from build123d import *

# Parameters (mm, degrees)
SKETCH1_W           = 10.53028371
SKETCH1_H           = 7.9375
BOSS_EXTRUDE1_DEPTH = 6.35
BOSS_EXTRUDE2_DEPTH = 11.1125
SKETCH3_R           = 0.75
BOSS_EXTRUDE3_DEPTH = 3.5


with BuildPart() as part:
    # Sketch1 → Boss-Extrude1 (new body)
    with BuildSketch(Plane(origin=(0, 0, 0), x_dir=(1, 0, 0), z_dir=(0, 1, 0))):
        with BuildLine():
            Line((-5.265141855, 0), (-5.265141855, 7.9375))
            ThreePointArc((-5.265141855, 7.9375), (-8.392737967, 4.504173), (-9.525, 0))
            Line((-9.525, 0), (-5.265141855, 0))
        make_face()
        with BuildLine():
            Line((-5.265141855, -7.9375), (-5.265141855, 0))
            Line((-5.265141855, 0), (-9.525, 0))
            ThreePointArc((-9.525, 0), (-8.392737967, -4.504173), (-5.265141855, -7.9375))
        make_face()
        with Locations((0, -3.96875)):
            Rectangle(SKETCH1_W, SKETCH1_H)
        with BuildLine():
            ThreePointArc((9.525, 0), (8.392737967, 4.504173), (5.265141855, 7.9375))
            Line((5.265141855, 7.9375), (5.265141855, 0))
            Line((5.265141855, 0), (9.525, 0))
        make_face()
        with BuildLine():
            Line((9.525, 0), (5.265141855, 0))
            Line((5.265141855, 0), (5.265141855, -7.9375))
            ThreePointArc((5.265141855, -7.9375), (8.392737967, -4.504173), (9.525, 0))
        make_face()
        with Locations((0, 3.96875)):
            Rectangle(SKETCH1_W, SKETCH1_H)
    extrude(amount=BOSS_EXTRUDE1_DEPTH)

    # Sketch2 → Boss-Extrude2 (add)
    with BuildSketch(Plane(origin=(0, 6.35, 0), x_dir=(1, 0, 0), z_dir=(0, 1, 0))):
        with BuildLine():
            Line((5.265141855, 7.9375), (-5.265141855, 7.9375))
            ThreePointArc((-5.265141855, 7.9375), (-9.525, 0), (-5.265141855, -7.9375))
            Line((-5.265141855, -7.9375), (5.265141855, -7.9375))
            ThreePointArc((5.265141855, -7.9375), (9.525, 0), (5.265141855, 7.9375))
        make_face()
    extrude(amount=BOSS_EXTRUDE2_DEPTH)

    # Sketch3 → Boss-Extrude3 (add)
    with BuildSketch(Plane(origin=(0, 17.4625, 0), x_dir=(1, 0, 0), z_dir=(0, 1, 0))):
        Circle(SKETCH3_R)
    extrude(amount=BOSS_EXTRUDE3_DEPTH)


solid = part.part
Work out the finished part from the listing and answer in its coordinate system (mm). A direction names the side the tool comes from. Coordinates: 2 decimals unless noted, no trailing zeros. Loops run counter-clockwise (first coordinate to the right, second up) from the corner with the lowest first, then second, coordinate; pieces in that order, holes last. Notation, with made-up numbers: M 81,0 L 131,0 A18 cw 131,8 Z; hole C -30,9 d1. An arc over 180 degrees is marked long. Answer in a Markdown table with one row per item. Add a question column.
1. Find section A-A, the plane x = 0. Write down the section's boundary in (y, z).
2. A tool of negligible diameter and unlimited length cuts with its end or side. For faces 1 (the flat face through (0, 20.962, 0)), 2 (the cylindrical face through (-0.75, 19.19, -0.03)), from which of +Z, -Z, +X, -X, +Y, -Y can it reach the whole face along a straight path? Write none if from no direction.
3. Consider L1, parallel to Y at x = -1.75, z = 5; L2, parallel to X at y = 14.75, z = -3.25; L3, parallel to Z at x = 8.75, y = 11. Determine where each line is inside the solid, lowest interval first.
4. Find section D-D, the plane x = 4.5. Write down the section's boundary in (y, z).
5. Find section C-C, the plane z = -1.75. Write down the section's boundary in (x, y), then the cut area to 3 significant figures.
6. Flat-ended cylindrical pins translate along their axes: P1, Ø5, axis at x = 4, z = -2.5, coming from the +Y side; P2, Ø2, axis at y = 11.5, z = -5, coming from the -X side; P3, Ø6, axis at y = 11, z = -5, coming from the +X side. Find the tip coordinate at first contact, or state that the pin passes through.
Reported:
| question | item | result |
|---|---|---|
| 1 | outline | M 0,-7.94 L 17.46,-7.94 L 17.46,-0.75 L 20.96,-0.75 L 20.96,0.75 L 17.46,0.75 L 17.46,7.94 L 0,7.94 Z |
| 2 | face 1 | +Z, -Z, +X, -X, +Y |
| 2 | face 2 | +Y |
| 3 | L1 | y = 0 to 17.46 |
| 3 | L2 | x = -8.95 to 8.95 |
| 3 | L3 | z = -3.76 to 3.76 |
| 4 | outline | M 0,-7.94 L 17.46,-7.94 L 17.46,7.94 L 0,7.94 Z |
| 5 | outline | M -9.36,0 L 9.36,0 L 9.36,17.46 L -9.36,17.46 Z |
| 5 | area | 327 mm^2 |
| 6 | P1 | stops at y = 17.46 |
| 6 | P2 | stops at x = -8.64 |
| 6 | P3 | stops at x = 9.31 |
